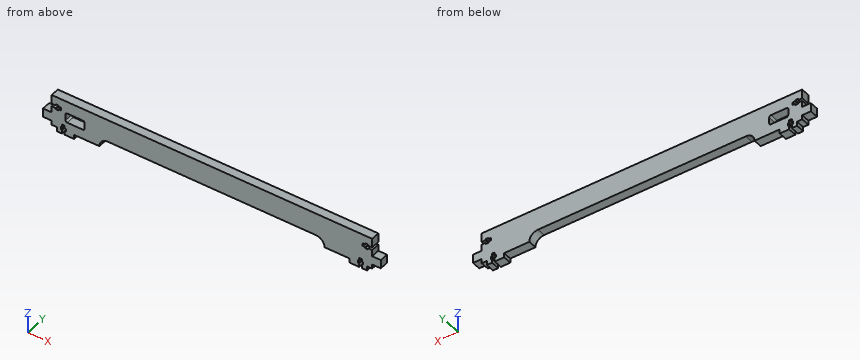
```python
from build123d import *

# Parameters (mm, degrees)
MAINSHAPE_DEPTH      = 10
SKETCH15_W           = 20
SKETCH15_H           = 10
BOSS_EXTRUDE4_DEPTH  = 10
SCREWSLOTS_DEPTH     = 197.606205395
LCDCABLECUTOUT_DEPTH = 197.606205395
CUT_EXTRUDE5_DEPTH   = 197.606205395


with BuildPart() as part:
    # Sketch1 → MainShape (new body)
    with BuildSketch(Plane(origin=(0, 0, 0), x_dir=(1, 0, 0), z_dir=(0, 1, 0))):
        Polygon((-185, 18), (0, 18), (0, -18), (-185, -18), (-185, 3), (-195, 3), (-195, 13), (-185, 13), align=None)
    mainshape = extrude(amount=MAINSHAPE_DEPTH)

    # Sketch15 → Boss-Extrude4 (add, through all)
    with BuildSketch(Plane(origin=(0, 10, 0), x_dir=(1, 0, 0), z_dir=(0, 1, 0))):
        with Locations((-169.1, 18)):
            Rectangle(SKETCH15_W, SKETCH15_H)
    boss_extrude4 = extrude(amount=-BOSS_EXTRUDE4_DEPTH)

    # Sketch2 → ScrewSlots (cut, through all)
    with BuildSketch(Plane(origin=(0, 10, 0), x_dir=(1, 0, 0), z_dir=(0, 1, 0))):
        with BuildLine():
            Line((-173.05, 23), (-173.05, 18.5))
            Line((-173.05, 18.5), (-173.85, 18.5))
            ThreePointArc((-173.85, 18.5), (-174.203553391, 18.353553391), (-174.35, 18))
            Line((-174.35, 18), (-174.35, 15.5))
            ThreePointArc((-174.35, 15.5), (-174.203553391, 15.146446609), (-173.85, 15))
            Line((-173.85, 15), (-173.05, 15))
            Line((-173.05, 15), (-173.05, 12))
            Line((-173.05, 12), (-169.95, 12))
            Line((-169.95, 12), (-169.95, 15))
            Line((-169.95, 15), (-169.15, 15))
            ThreePointArc((-169.15, 15), (-168.796446609, 15.146446609), (-168.65, 15.5))
            Line((-168.65, 15.5), (-168.65, 18))
            ThreePointArc((-168.65, 18), (-168.796446609, 18.353553391), (-169.15, 18.5))
            Line((-169.15, 18.5), (-169.95, 18.5))
            Line((-169.95, 18.5), (-169.95, 23))
            Line((-169.95, 23), (-173.05, 23))
        make_face()
        with BuildLine():
            Line((-174, -7.55), (-174, -4.45))
            Line((-174, -4.45), (-177, -4.45))
            Line((-177, -4.45), (-177, -3.5))
            ThreePointArc((-177, -3.5), (-177.146446609, -3.146446609), (-177.5, -3))
            Line((-177.5, -3), (-180, -3))
            ThreePointArc((-180, -3), (-180.353553391, -3.146446609), (-180.5, -3.5))
            Line((-180.5, -3.5), (-180.5, -4.45))
            Line((-180.5, -4.45), (-185, -4.45))
            Line((-185, -4.45), (-185, -7.55))
            Line((-185, -7.55), (-180.5, -7.55))
            Line((-180.5, -7.55), (-180.5, -8.5))
            ThreePointArc((-180.5, -8.5), (-180.353553391, -8.853553391), (-180, -9))
            Line((-180, -9), (-177.5, -9))
            ThreePointArc((-177.5, -9), (-177.146446609, -8.853553391), (-177, -8.5))
            Line((-177, -8.5), (-177, -7.55))
            Line((-177, -7.55), (-174, -7.55))
        make_face()
    screwslots = extrude(amount=-SCREWSLOTS_DEPTH, mode=Mode.SUBTRACT)

    # Mirror1: MainShape, Boss-Extrude4, ScrewSlots across plane
    add(mainshape.mirror(Plane(origin=(0, 0, 0), x_dir=(0, 0, 1), z_dir=(1, 0, 0))))
    add(boss_extrude4.mirror(Plane(origin=(0, 0, 0), x_dir=(0, 0, 1), z_dir=(1, 0, 0))))
    add(screwslots.mirror(Plane(origin=(0, 0, 0), x_dir=(0, 0, 1), z_dir=(1, 0, 0))), mode=Mode.SUBTRACT)

    # Sketch11 → LCDCableCutout (cut, through all)
    with BuildSketch(Plane.XZ):
        with BuildLine():
            Line((-149, -7), (-167, -7))
            ThreePointArc((-167, -7), (-168.414213562, -6.414213562), (-169, -5))
            Line((-169, -5), (-169, 2))
            ThreePointArc((-169, 2), (-168.414213562, 3.414213562), (-167, 4))
            Line((-167, 4), (-149, 4))
            ThreePointArc((-149, 4), (-147.585786438, 3.414213562), (-147, 2))
            Line((-147, 2), (-147, -5))
            ThreePointArc((-147, -5), (-147.585786438, -6.414213562), (-149, -7))
        make_face()
    extrude(amount=-LCDCABLECUTOUT_DEPTH, mode=Mode.SUBTRACT)

    # Sketch13 → Cut-Extrude5 (cut, through all)
    with BuildSketch(Plane(origin=(0, 10, 0), x_dir=(1, 0, 0), z_dir=(0, 1, 0))):
        with BuildLine():
            Line((120, 8), (-120, 8))
            ThreePointArc((-120, 8), (-130, 18), (-120, 28))
            Line((-120, 28), (120, 28))
            ThreePointArc((120, 28), (130, 18), (120, 8))
        make_face()
    extrude(amount=-CUT_EXTRUDE5_DEPTH, mode=Mode.SUBTRACT)


solid = part.part
```
Geometry: final body of the model. Coordinates: model frame, mm. Round coordinates to 2 decimals unless told otherwise and drop trailing zeros. Loops run counter-clockwise (first coordinate to the right, second up) from the corner with the lowest first, then second, coordinate; pieces in that order, holes last. Notation, with made-up numbers: (-32, 61.25) -> (13, 61.25) arc R23 cw to (13, 80.25) -> close; hole circle Ø5 at (22, 58). An arc over 180 degrees is marked (long way). Use one line per item in the form item = value. Start each with the question number.
1) Section B-B on x = 104. Output: boundary loops of the cut face in (y, z).
2) First-contact query: P1, Ø1.5, axis at y = 5.5, z = -21, coming from the -X side; P2, Ø4, axis at x = 101, y = 6, coming from the -Z side; P3, Ø2, axis at y = 6, z = -16.5, coming from the -X side. Flat tips, straight axial feed; report the tip coordinate or a pass-through.
3) Section A-A on x = -153. Output: boundary loops of the cut face in (y, z).
4) Line query: L1, parallel to X at y = 1.5, z = -21; L2, parallel to Z at x = -157, y = 6.5; L3, parallel to X at y = 2.25, z = -12.5. Output: solid intervals per line, ascending.
Response:
q1.outline = (0, -8) -> (10, -8) -> (10, 18) -> (0, 18) -> close
q2.P1 = -179.1
q2.P2 = -8
q2.P3 = -185
q3.outline = (0, -18) -> (10, -18) -> (10, -7) -> (0, -7) -> close; (0, 4) -> (10, 4) -> (10, 18) -> (0, 18) -> close
q4.L1 = -179.1 to -173.05, -169.95 to -159.1, 159.1 to 169.95, 173.05 to 179.1
q4.L2 = -18 to -7, 4 to 18
q4.L3 = -195 to -173.05, -169.95 to -128.35, 128.35 to 169.95, 173.05 to 195
